Part print with two shaded views. Sizes in mm from the minimum x, y, z corner. A direction names the side the tool comes from. Round coordinates to 2 decimals unless told otherwise and drop trailing zeros. Order: outer loops, then holes, each group sorted by start corner. A loop starts at its lowest first (then second) coordinate and runs counter-clockwise, first axis right, second up. Notation, with made-up numbers: M -9,-35.5 L -4,-35.5 A12 ccw -4,-14.5 Z; hole C 27.5,68 d8. An arc over 180 degrees is marked long. One line per question, with ' | ' between items.
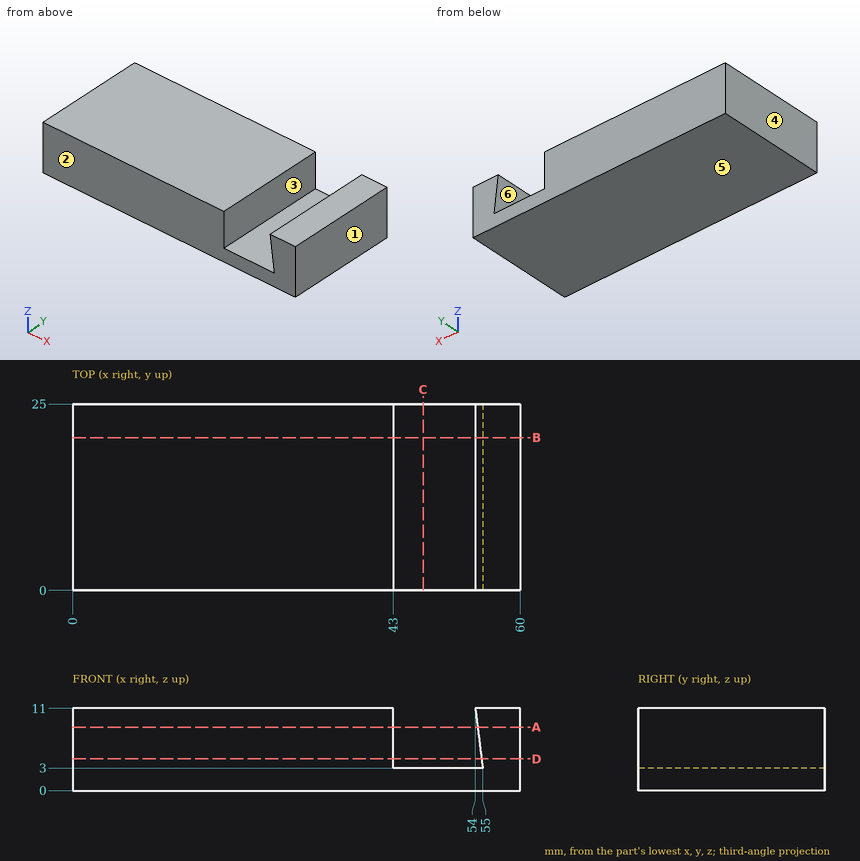
1) Probe line 1 (Z direction, x = 47.5, y = 22.5); line 2 (X direction, y = 15.5, z = 10) (3 decimals); line 3 (X direction, y = 1.75, z = 9.75). List the from-to ranges inside material, lowest first. Write a range as [from, to].
The answers:
line 1: z = [0, 3] | line 2: x = [0, 43], [54.125, 60] | line 3: x = [0, 43], [54.16, 60]
2) Saw through at A-A (z = 8.5). List the corners of the cut face in (x, y).
The answers:
outline: M 0,0 L 43,0 L 43,25 L 0,25 Z; M 54.31,0 L 60,0 L 60,25 L 54.31,25 Z
3) Saw through at C-C (x = 47). List the corners of the cut face in (y, z).
The answers:
outline: M 0,0 L 25,0 L 25,3 L 0,3 Z
4) Drop a flat-ended pin along its axis: pin 1 (6 mm diameter, centred on x = 47.5, y = 10, fed in from +Z). Give the stop position or say it passes through.
The answers:
pin 1: stops at z = 3
5) Saw through at D-D (z = 4.25). List the corners of the cut face in (x, y).
The answers:
outline: M 0,0 L 43,0 L 43,25 L 0,25 Z; M 54.84,0 L 60,0 L 60,25 L 54.84,25 Z
6) Which spindle directions (+Z, -Z, +X, -X, +Y, -Y) get a long thin tool onto all of the face, cutting with end or side? Do the marked faces 5 and 6. Say none if no direction does.
The answers:
face 5: -Z, +X, -X, +Y, -Y | face 6: +Y, -Y
7) Saw through at B-B (y = 20.5). List the corners of the cut face in (x, z).
The answers:
outline: M 0,0 L 60,0 L 60,11 L 54,11 L 55,3 L 43,3 L 43,11 L 0,11 Z
8) Two-plate mould, pull along X, no slides. Class the marked faces 1, 2, 3 and 4: released by +X, released by -X, zero draft, split by the parting line, or undercut.
The answers:
face 1: released by +X | face 2: zero draft | face 3: undercut | face 4: released by -X
